```python
from build123d import *

# Parameters (mm, degrees)
SKETCH1_W           = 150
SKETCH1_H           = 30
BOSS_EXTRUDE1_DEPTH = 5
SKETCH2_R           = 2.15
CUT_EXTRUDE1_DEPTH  = 6
SKETCH3_W           = 10
SKETCH3_H           = 135
BOSS_EXTRUDE2_DEPTH = 10
BOSS_EXTRUDE3_DEPTH = 10
SKETCH6_W           = 20
SKETCH6_H           = 10
BOSS_EXTRUDE4_DEPTH = 65
SKETCH5_R           = 2.65
CUT_EXTRUDE3_DEPTH  = 10
BOSS_EXTRUDE5_REACH = 109.5
SKETCH7_W           = 5.3
SKETCH7_H           = 10
FILLET1_R           = 3
FILLET2_R           = 3


with BuildPart() as part:
    # Sketch1 → Boss-Extrude1 (new body)
    with BuildSketch(Plane.XY):
        with Locations((75, 15)):
            Rectangle(SKETCH1_W, SKETCH1_H)
    extrude(amount=BOSS_EXTRUDE1_DEPTH)

    # Sketch2 → Cut-Extrude1 (cut, through all)
    with BuildSketch(Plane.XY.offset(5)):
        with Locations((75, 20)):
            Circle(SKETCH2_R)
        with Locations((55, 20)):
            Circle(SKETCH2_R)
        with Locations((95, 20)):
            Circle(SKETCH2_R)
    extrude(amount=-CUT_EXTRUDE1_DEPTH, mode=Mode.SUBTRACT)

    # Sketch3 → Boss-Extrude2 (add)
    with BuildSketch(Plane(origin=(0, 30, 0), x_dir=(1, 0, 0), z_dir=(0, 1, 0))):
        with Locations((112.5, 67.5)):
            Rectangle(SKETCH3_W, SKETCH3_H)
        with Locations((37.5, 67.5)):
            Rectangle(SKETCH3_W, SKETCH3_H)
    extrude(amount=-BOSS_EXTRUDE2_DEPTH)

    # Sketch4 → Boss-Extrude3 (add)
    with BuildSketch(Plane(origin=(0, 30, 0), x_dir=(1, 0, 0), z_dir=(0, 1, 0))):
        Polygon((32.5, 67.5), (32.5, 112.5), (7.5, 0), (17.5, 0), align=None)
        Polygon((117.5, 112.5), (117.5, 67.5), (132.5, 0), (142.5, 0), align=None)
    extrude(amount=-BOSS_EXTRUDE3_DEPTH)

    # Sketch6 → Boss-Extrude4 (add)
    with BuildSketch(Plane.ZY.offset(-107.5)):
        with Locations((-80, 25)):
            Rectangle(SKETCH6_W, SKETCH6_H)
    extrude(amount=BOSS_EXTRUDE4_DEPTH)

    # Sketch5 → Cut-Extrude3 (cut)
    with BuildSketch(Plane(origin=(0, 30, 0), x_dir=(1, 0, 0), z_dir=(0, 1, 0))):
        with Locations((37.5, 48)):
            Circle(SKETCH5_R)
        with Locations((112.5, 48)):
            Circle(SKETCH5_R)
        with Locations((112.5, 123)):
            Circle(SKETCH5_R)
        with Locations((37.5, 123)):
            Circle(SKETCH5_R)
    extrude(amount=-CUT_EXTRUDE3_DEPTH, mode=Mode.SUBTRACT)

    # Sketch7 → Boss-Extrude5 (add, up to next)
    with BuildSketch(Plane.ZY.offset(-107.5), mode=Mode.PRIVATE) as boss_extrude5_sk1:
        with Locations((-123, 25)):
            Rectangle(SKETCH7_W, SKETCH7_H)
    boss_extrude5_tool1 = extrude(boss_extrude5_sk1.sketch, amount=BOSS_EXTRUDE5_REACH, mode=Mode.PRIVATE) - part.part
    add(boss_extrude5_tool1.solids().sort_by_distance((107.5, 25, -123))[0])

    # Fillet1
    fillet1_edges = [part.edges().sort_by_distance(p)[0] for p in [
        (42.5, 25, -125.65),
        (107.5, 25, -125.65),
        (32.5, 25, -135),
        (42.5, 25, -135),
        (42.5, 25, 0),
        (32.5, 25, 0),
        (117.5, 25, 0),
        (107.5, 25, 0),
        (107.5, 25, -135),
        (117.5, 25, -135),
        (32.5, 25, -67.5),
        (32.5, 25, -112.5),
        (7.5, 25, 0),
        (17.5, 25, 0),
        (117.5, 25, -112.5),
        (142.5, 25, 0),
        (132.5, 25, 0),
        (117.5, 25, -67.5),
        (42.5, 25, -70),
        (107.5, 25, -70),
    ]]
    fillet(fillet1_edges, radius=FILLET1_R)

    # Fillet2
    fillet2_edges = [part.edges().sort_by_distance(p)[0] for p in [
        (42.5, 25, -120.35),
        (107.5, 25, -120.35),
        (42.5, 25, -90),
        (107.5, 25, -90),
    ]]
    fillet(fillet2_edges, radius=FILLET2_R)


solid = part.part
```
Here's how the part is built. I have some questions about the finished solid (model axes, mm). A direction names the side the tool comes from. Coordinates: 2 decimals unless noted, no trailing zeros. Loops run counter-clockwise (first coordinate to the right, second up) from the corner with the lowest first, then second, coordinate; pieces in that order, holes last. Notation, with made-up numbers: (-11, 52.5) -> (47, 52.5) arc R9 ccw to (47, 60.5) -> close; hole circle Ø3 at (89, 59.25). An arc over 180 degrees is marked (long way). Return JSON: item names as keys, results as strings.
1) Thinking about a two-plate mould opening in X: for faces 1 (the face through (75, 25, -120.35)), 2 (the face through (32.5, 25, -122)), 3 (the face through (150, 15, 2)), 4 (the face through (75, 30, -71)), which applies, +X half, -X half, draft (parallel to the pull), parting line (faces both ways), or undercut?
Results below:
{"face 1": "undercut", "face 2": "-X half", "face 3": "+X half", "face 4": "draft"}
2) I need wall thicknesses on line 1 (Z direction, x = 112.5, y = 25); line 2 (X direction, y = 23.25, z = -123); line 3 (Z direction, x = 60, y = 24). Which ranges of each line are inside material? Lowest first, please. Write a range as from..to.
Results below:
{"line 1": "-135..-125.65, -120.35..-50.65, -45.35..5", "line 2": "32.5..34.85, 40.15..109.85, 115.15..117.5", "line 3": "-125.65..-120.35, -90..-70, 0..5"}
3) If we section it at C-C, the plane x = 75: Write out the boundary of the cut face in (y, z).
Results below:
{"outline": "(0, 0) -> (17.85, 0) -> (17.85, 5) -> (0, 5) -> close; (20, -125.65) -> (30, -125.65) -> (30, -120.35) -> (20, -120.35) -> close; (20, -90) -> (30, -90) -> (30, -70) -> (20, -70) -> close; (22.15, 0) -> (30, 0) -> (30, 5) -> (22.15, 5) -> close"}
4) For faces 5 (the face through (69, 20, -73)), 6 (the face through (37, 25, -135)), 7 (the face through (32.5, 25, -21)), 8 (the face through (73.294, 18.692, 2.535)), 9 (the face through (42.5, 25, -130)), which set-ups out of +Z, -Z, +X, -X, +Y, -Y let a thin tool reach every point of the face, with its end or its side?
Results below:
{"face 5": "-Z, +X, -X, -Y", "face 6": "-Z, +X, -X, +Y, -Y", "face 7": "+Y, -Y", "face 8": "+Z", "face 9": "-Z, +Y, -Y"}
5) If we section it at A-A, the plane z = -123: Write out the boundary of the cut face in (x, y), then the cut area to 3 significant figures.
Results below:
{"outline": "(32.5, 20) -> (34.85, 20) -> (34.85, 30) -> (32.5, 30) -> close; (40.15, 20) -> (109.85, 20) -> (109.85, 30) -> (40.15, 30) -> close; (115.15, 20) -> (117.5, 20) -> (117.5, 30) -> (115.15, 30) -> close", "area": "744 mm²"}
6) Will these pins go through, and if not, where does the flat tip stop? pin 1 (4 mm diameter, centred on y = 23.5, z = -108, fed in from +X); pin 2 (8 mm diameter, centred on x = 21, y = 11.5, fed in from -Z); pin 3 (3 mm diameter, centred on y = 25, z = -119.5, fed in from +X).
Results below:
{"pin 1": "x = 118.94", "pin 2": "z = 0", "pin 3": "x = 117.5"}
7) If we section it at B-B, the plane x = 50.5: Write out the boundary of the cut face in (y, z).
Results below:
{"outline": "(0, 0) -> (30, 0) -> (30, 5) -> (0, 5) -> close; (20, -125.65) -> (30, -125.65) -> (30, -120.35) -> (20, -120.35) -> close; (20, -90) -> (30, -90) -> (30, -70) -> (20, -70) -> close"}
8) If we section it at D-D, the plane z = -34: Write out the boundary of the cut face in (x, y), then the cut area to 3 significant figures.
Results below:
{"outline": "(15.06, 20) -> (25.06, 20) -> (25.06, 30) -> (15.06, 30) -> close; (32.5, 20) -> (42.5, 20) -> (42.5, 30) -> (32.5, 30) -> close; (107.5, 20) -> (117.5, 20) -> (117.5, 30) -> (107.5, 30) -> close; (124.94, 20) -> (134.94, 20) -> (134.94, 30) -> (124.94, 30) -> close", "area": "400 mm²"}
